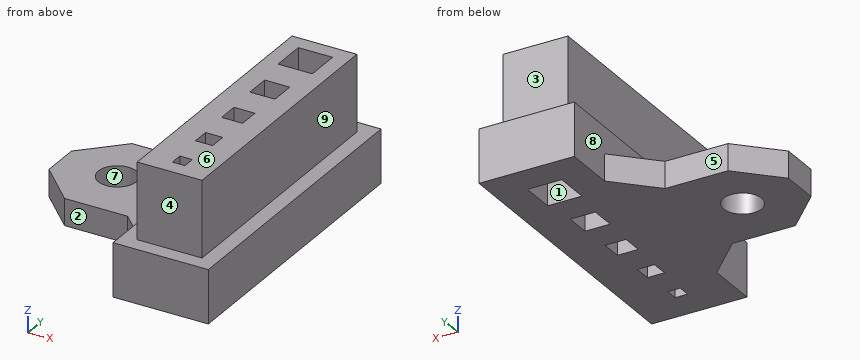
from build123d import *

# Parameters (mm, degrees)
F0_W     = 1.65
F0_H     = 1.65
F0_W_2   = 2.25
F0_H_2   = 2.25
F0_W_3   = 2.75
F0_H_3   = 2.75
F0_R     = 2.5
F0_W_4   = 3.3
F0_H_4   = 3.3
F0_W_5   = 4.5
F0_H_5   = 4.5
F1_DEPTH = 3.5
F2_W     = 1.65
F2_H     = 1.65
F2_W_2   = 2.25
F2_H_2   = 2.25
F2_W_3   = 2.75
F2_H_3   = 2.75
F2_W_4   = 3.3
F2_H_4   = 3.3
F2_W_5   = 4.5
F2_H_5   = 4.5
F3_DEPTH = 3.5
F4_W     = 8.5
F4_H     = 34.45
F5_DEPTH = 10
F6_SIZE  = 5


with BuildPart() as f1:
    # F0 (on Top) → F1 (new body)
    with BuildSketch(Plane.XY):
        Polygon((12.5, 19.225), (0, 19.225), (0, 7.5), (-18.25, 7.5), (-18.25, -7.5), (0, -7.5), (0, -19.225), (12.5, -19.225), align=None)
        with Locations((6.25, -14.4)):
            Rectangle(F0_W, F0_H, mode=Mode.SUBTRACT)
        with Locations((6.25, -8.45)):
            Rectangle(F0_W_2, F0_H_2, mode=Mode.SUBTRACT)
        with Locations((6.25, -1.95)):
            Rectangle(F0_W_3, F0_H_3, mode=Mode.SUBTRACT)
        with Locations((-10.75, 0)):
            Circle(F0_R, mode=Mode.SUBTRACT)
        with Locations((6.25, 5.075)):
            Rectangle(F0_W_4, F0_H_4, mode=Mode.SUBTRACT)
        with Locations((6.25, 12.975)):
            Rectangle(F0_W_5, F0_H_5, mode=Mode.SUBTRACT)
    extrude(amount=F1_DEPTH)

    # F2 (on face) → F3 (join)
    with BuildSketch(Plane.XY.offset(3.5)):
        Polygon((12.5, 19.225), (0, 19.225), (0, 7.5), (0, -7.5), (0, -19.225), (12.5, -19.225), align=None)
        with Locations((6.25, -14.4)):
            Rectangle(F2_W, F2_H, mode=Mode.SUBTRACT)
        with Locations((6.25, -8.45)):
            Rectangle(F2_W_2, F2_H_2, mode=Mode.SUBTRACT)
        with Locations((6.25, -1.95)):
            Rectangle(F2_W_3, F2_H_3, mode=Mode.SUBTRACT)
        with Locations((6.25, 5.075)):
            Rectangle(F2_W_4, F2_H_4, mode=Mode.SUBTRACT)
        with Locations((6.25, 12.975)):
            Rectangle(F2_W_5, F2_H_5, mode=Mode.SUBTRACT)
    extrude(amount=F3_DEPTH)

    # F4 (on face) → F5 (join)
    with BuildSketch(Plane.XY.offset(7)):
        with Locations((6.25, 0)):
            Rectangle(F4_W, F4_H)
        Polygon((5.425, -13.575), (6.75, -13.575), (7.075, -13.575), (7.075, -14.5), (7.075, -15.225), (6.75, -15.225), (5.425, -15.225), (5.425, -14.5), align=None, mode=Mode.SUBTRACT)
        Polygon((5.125, -7.325), (7, -7.325), (7.375, -7.325), (7.375, -9), (7.375, -9.575), (7, -9.575), (5.125, -9.575), (5.125, -9), align=None, mode=Mode.SUBTRACT)
        Polygon((4.875, -0.575), (7.25, -0.575), (7.625, -0.575), (7.625, -3), (7.625, -3.325), (7.25, -3.325), (4.875, -3.325), (4.875, -3), align=None, mode=Mode.SUBTRACT)
        Polygon((4.6, 6.725), (7.5, 6.725), (7.9, 6.725), (7.9, 6.5), (7.9, 3.5), (7.9, 3.425), (7.5, 3.425), (4.6, 3.425), (4.6, 3.5), (4.6, 6.5), align=None, mode=Mode.SUBTRACT)
        Polygon((8, 10.725), (4, 10.725), (4, 14.5), (4, 15.225), (8, 15.225), (8.5, 15.225), (8.5, 14.5), (8.5, 10.725), align=None, mode=Mode.SUBTRACT)
    extrude(amount=F5_DEPTH)

    # F6
    f6_edges = [f1.edges().sort_by_distance(p)[0] for p in [
        (0, 7.5, 1.75),
        (0, -7.5, 1.75),
        (-18.25, -7.5, 1.75),
        (-18.25, 7.5, 1.75),
    ]]
    chamfer(f6_edges, length=F6_SIZE)


solid = f1.part
Work out the finished part from the listing and answer in its coordinate system (mm). Face numbers are marked on the shaded views. A direction names the side the tool comes from. Round coordinates to 2 decimals unless told otherwise and drop trailing zeros. Order: outer loops, then holes, each group sorted by start corner. A loop starts at its lowest first (then second) coordinate and runs counter-clockwise, first axis right, second up. Notation, with made-up numbers: M 8.25,-39 L 15.25,-39 A13 cw 15.25,-31 Z; hole C -9.5,-16 d11. An arc over 180 degrees is marked long. Put each result on its own line as item: value. Start each with the question number.
Q1. Section D-D, the plane z = 15.25 is taken. Write down the section's boundary in (x, y) (3 decimals).
Q2. A tool of negligible diameter and unlimited length cuts with its end or side. For the marked faces 1, 2, 3, 4 and 5, from which of +Z, -Z, +X, -X, +Y, -Y can it reach the whole face along a straight path? Write none if from no direction.
Q3. Straight lines are drawn through the part: L1, parallel to X at y = 14, z = 4.25; L2, parallel to X at y = -9, z = 15.5 (3 decimals); L3, parallel to Y at x = -10.75, z = 1.05. For each, find the intervals that lie inside material, in ascending order. Write a range as [from, to].
Q4. Section B-B, the plane x = -10.75 is taken. Write down the section's boundary in (y, z).
Q5. Flat-ended cylindrical pins translate along their axes: pin 1 (1.3 mm diameter, centred on y = -14.5, z = 9.5, fed in from -X); pin 2 (2 mm diameter, centred on y = -7, z = 4, fed in from -X); pin 3 (5 mm diameter, centred on x = 2.5, z = 11.5, fed in from +Y) (3 decimals). Find the tip coordinate at first contact, or state that the pin passes through.
Q6. Section C-C, the plane x = 9 is taken. Write down the section's boundary in (y, z) (3 decimals).
Q7. For a pull along X with two mould halves and no side action, classify the marked faces 6, 7, 8 and 9 as pulls with the +X half, pulls with the -X half, needs draft (parallel to the pull), parting line crosses it, or undercut.
Q8. Section A-A, the plane y = 0 is taken. Write down the section's boundary in (x, z).
Findings below:
1. outline: M 2,-17.225 L 10.5,-17.225 L 10.5,17.225 L 2,17.225 Z; hole M 4,10.725 L 8.5,10.725 L 8.5,15.225 L 4,15.225 Z; hole M 4.6,3.425 L 7.9,3.425 L 7.9,6.725 L 4.6,6.725 Z; hole M 4.875,-3.325 L 7.625,-3.325 L 7.625,-0.575 L 4.875,-0.575 Z; hole M 5.125,-9.575 L 7.375,-9.575 L 7.375,-7.325 L 5.125,-7.325 Z; hole M 5.425,-15.225 L 7.075,-15.225 L 7.075,-13.575 L 5.425,-13.575 Z
2. face 1: +Z, -Z
2. face 2: +Z, -Z, -X, -Y
2. face 3: +Z, +X, -X, +Y
2. face 4: +Z, +X, -X, -Y
2. face 5: +Z, -Z, -X, +Y
3. L1: x = [0, 4], [8.5, 12.5]
3. L2: x = [2, 5.125], [7.375, 10.5]
3. L3: y = [-7.5, -2.5], [2.5, 7.5]
4. outline: M -7.5,0 L -2.5,0 L -2.5,3.5 L -7.5,3.5 Z; M 2.5,0 L 7.5,0 L 7.5,3.5 L 2.5,3.5 Z
5. pin 1: stops at x = 2
5. pin 2: stops at x = -14.62
5. pin 3: stops at y = 17.225
6. outline: M -19.225,0 L 19.225,0 L 19.225,7 L 17.225,7 L 17.225,17 L -17.225,17 L -17.225,7 L -19.225,7 Z
7. face 6: needs draft
7. face 7: undercut
7. face 8: pulls with the -X half
7. face 9: pulls with the +X half
8. outline: M -18.25,0 L -13.25,0 L -13.25,3.5 L -18.25,3.5 Z; M -8.25,0 L 12.5,0 L 12.5,7 L 10.5,7 L 10.5,17 L 2,17 L 2,7 L 0,7 L 0,3.5 L -8.25,3.5 Z
